```python
from build123d import *

# Parameters (mm, degrees)
SKETCH_1_R          = 1.6
EXTRUDE_1_DEPTH     = 1.6
SKETCH_3_R          = 0.8
EXTRUDE_3_DEPTH     = 5.5
CUT_EXTRUDE_1_DEPTH = 0.8


with BuildPart() as part:
    # 草图1 → 凸台-拉伸1 (new body)
    with BuildSketch(Plane.XY):
        Circle(SKETCH_1_R)
    extrude(amount=EXTRUDE_1_DEPTH)

    # 草图3 → 凸台-拉伸3 (add)
    with BuildSketch(Plane.XY):
        Circle(SKETCH_3_R)
    extrude(amount=-EXTRUDE_3_DEPTH)

    # 草图4 → 切除-拉伸1 (cut)
    with BuildSketch(Plane.XY.offset(1.6)):
        Polygon((0.8, 0), (0.4, 0.692820323), (-0.4, 0.692820323), (-0.8, 0), (-0.4, -0.692820323), (0.4, -0.692820323), align=None)
    extrude(amount=-CUT_EXTRUDE_1_DEPTH, mode=Mode.SUBTRACT)


solid = part.part
```
Input: part model. Units: mm. Frame: model coordinates. A direction names the side the tool comes from. Give positions to 0.01 mm unless a question says otherwise; leave off trailing zeros. Write each loop counter-clockwise with the first axis right and the second up, starting at its lowest first coordinate (ties: lowest second). Pieces come first, ordered by that corner, then holes. Notation, with made-up numbers: (26.25, 6.25) - (75.25, 6.25) arc R24 ccw to (75.25, 40.25) - close; hole circle Ø3 at (31.5, 4). An arc over 180 degrees is marked (long way). Write item = value, one per line. Start each with the question number.
1) Cut plane D-D (z = -1). Return loops of the section in (x, y).
2) Pin query (flat end, axial travel): pin 1 (1 mm diameter, centred on y = 0, z = -2.5, fed in from +X). Return the tip coordinate at first contact, or that it passes through.
3) Cut plane B-B (x = 0). Return loops of the section in (y, z), and give its area (3 significant figures).
4) Cut plane C-C (y = -0.6). Return loops of the section in (x, z), and give its area (3 significant figures).
5) Material intervals for L1, parallel to Z at x = -0.35, y = 1.2; L2, parallel to X at y = 0.05, z = -3; L3, parallel to Z at x = 0.25, y = -0.3, sorted ascending. Write a range as [from, to].
6) Cut plane A-A (z = 1). Return loops of the section in (x, y).
7) Reachability of faces 1 (the face through (0, 0, -5.5)), 2 (the face through (0, 1, 0)) from +Z, -Z, +X, -X, +Y, -Y: full face, straight path, thin tool, end or side. Return the list, or none.
8) Draft query along X for faces 3 (the face through (-1.27, -0.97, 0.79)), 4 (the face through (0, 1, 1.6)), 5 (the face through (0, 0, 0.8)). Return one class per face: pulls with the +X half, pulls with the -X half, needs draft (parallel to the pull), parting line crosses it, or undercut.
Answers follow:
q1.outline = circle Ø1.6 at (0, 0)
q2.pin_1 = 0.8
q3.outline = (-1.6, 0) - (-0.8, 0) - (-0.8, -5.5) - (0.8, -5.5) - (0.8, 0) - (1.6, 0) - (1.6, 1.6) - (0.69, 1.6) - (0.69, 0.8) - (-0.69, 0.8) - (-0.69, 1.6) - (-1.6, 1.6) - close
q3.area = 12.8 mm^2
q4.outline = (-1.48, 0) - (-0.53, 0) - (-0.53, -5.5) - (0.53, -5.5) - (0.53, 0) - (1.48, 0) - (1.48, 1.6) - (0.45, 1.6) - (0.45, 0.8) - (-0.45, 0.8) - (-0.45, 1.6) - (-1.48, 1.6) - close
q4.area = 9.84 mm^2
q5.L1 = [0, 1.6]
q5.L2 = [-0.8, 0.8]
q5.L3 = [-5.5, 0.8]
q6.outline = circle Ø3.2 at (0, 0); hole (-0.8, 0) - (-0.4, -0.69) - (0.4, -0.69) - (0.8, 0) - (0.4, 0.69) - (-0.4, 0.69) - close
q7.face_1 = -Z, +X, -X, +Y, -Y
q7.face_2 = -Z
q8.face_3 = parting line crosses it
q8.face_4 = needs draft
q8.face_5 = undercut
